Work out the finished part from the listing and answer in its coordinate system (mm). Face numbers are marked on the shaded views. A direction names the side the tool comes from. Round coordinates to 2 decimals unless told otherwise and drop trailing zeros. Loops run counter-clockwise (first coordinate to the right, second up) from the corner with the lowest first, then second, coordinate; pieces in that order, holes last. Notation, with made-up numbers: M 28.5,-11 L 67.5,-11 A24 ccw 67.5,21 Z; hole C -36,-35 d11. An arc over 180 degrees is marked long. One line per item, written item: value.
Autodesk Inventor part; units mm, degrees
ref_plane "YZ Plane" through (0, 0, 0) normal (1, 0, 0) x (0, 1, 0)
ref_plane "XZ Plane" through (0, 0, 0) normal (0, 1, 0) x (-1, 0, 0)
ref_plane "XY Plane" through (0, 0, 0) normal (0, 0, 1) x (1, 0, 0)
sketch "Sketch1" plane through (0, 0, 0) normal (0, 1, 0) x (-1, 0, 0)
  circle A0 centre (0, 0) radius 10
  circle A1 centre (0, 0) radius 8.6
extrude "Extrusion1" add sketch "Sketch1" along normal blind 5 contours A0 | A1
sketch "Sketch2" plane through (0, 0, 0) normal (0, -1, 0) x (1, 0, 0)
  circle A0 centre (0, 0) radius 8.6
  circle A1 centre (0, 0) radius 2.5
extrude "Extrusion2" add sketch "Sketch2" along normal blind 20 contours A0 | A1
sketch "Sketch3" plane through (0, -20, 0) normal (0, -1, 0) x (1, 0, 0)
  circle A0 centre (0, 0) radius 2.5
extrude "Extrusion3" cut sketch "Sketch3" against normal blind 10
sketch "Sketch4" plane through (0, 5, 0) normal (0, 1, 0) x (1, 0, 0)
  circle A0 centre (0, 0) radius 5
extrude "Extrusion4" add sketch "Sketch4" along normal blind 43
fillet "Fillet1" radius 2 1 edges at (-5, 48, 0)
properties part number "driven_shaft" material "Gold"
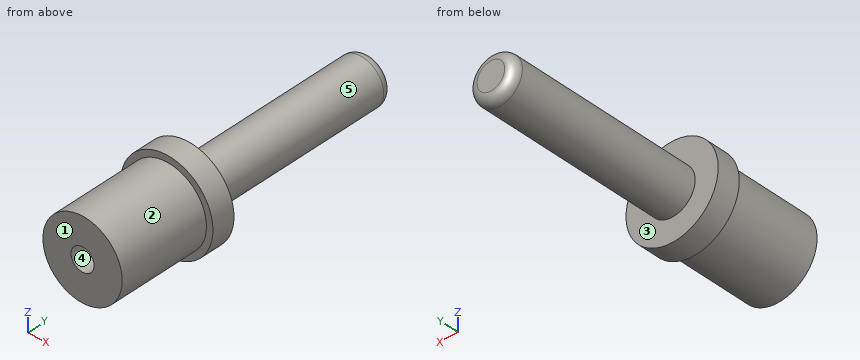
1) Find section A-A (z = 0). Give the vertices of the cut face in (x, y).
Check values:
outline: M -10,0 L -8.6,0 L -8.6,-20 L -2.5,-20 L -2.5,-10 L 2.5,-10 L 2.5,-20 L 8.6,-20 L 8.6,0 L 10,0 L 10,5 L 5,5 L 5,46 A2 ccw 3,48 L -3,48 A2 ccw -5,46 L -5,5 L -10,5 Z
2) Find section B-B (x = 0). Give the vertices of the cut face in (y, z).
Check values:
outline: M -20,-8.6 L 0,-8.6 L 0,-10 L 5,-10 L 5,-5 L 46,-5 A2 ccw 48,-3 L 48,3 A2 ccw 46,5 L 5,5 L 5,10 L 0,10 L 0,8.6 L -20,8.6 L -20,2.5 L -10,2.5 L -10,-2.5 L -20,-2.5 Z
3) For the marked faces 1 and 2, determine the directions among +Z, -Z, +X, -X, +Y, -Y from which every point of the face is accessible in a straight line to the end or side of a thin tool.
Check values:
face 1: +Z, -Z, +X, -X, -Y
face 2: -Y
4) The mould has two halves that part along X. Classify the marked faces 3, 4 and 5: +X half, -X half, draft (parallel to the pull), parting line (faces both ways), or undercut.
Check values:
face 3: draft
face 4: undercut
face 5: parting line
5) Each of these flat-tipped pins is pushed along its axis until it touches: pin 1 (1.5 mm diameter, centred on x = 1.5, y = 37.5, fed in from -Z); pin 2 (6 mm diameter, centred on y = 15, z = -3.5, fed in from -X); pin 3 (2 mm diameter, centred on x = -5.5, y = 14, fed in from -Z). Where does it stop, or does it pass through?
Check values:
pin 1: z = -4.94
pin 2: x = -4.97
pin 3: z = -2.18
6) Find section C-C (y = 12). Give the vertices of the cut face in (x, z), then the cut area to 3 significant figures.
Check values:
outline: C 0,0 d10
area: 78.5 mm2
7) Find section D-D (z = -5.75). Give the vertices of the cut face in (x, y).
Check values:
outline: M -8.18,0 L -6.4,0 L -6.4,-20 L 6.4,-20 L 6.4,0 L 8.18,0 L 8.18,5 L -8.18,5 Z
8) Find the intervals of material crossed by probe 1 along Z at (x, y) = (0, -15.5); probe 2 along Y at (x, z) = (0.75, 1.25); probe 3 along Y at (x, z) = (8, 3.5), in increasing order. Write a range as from..to.
Check values:
probe 1: -8.6..-2.5, 2.5..8.6
probe 2: -10..48
probe 3: 0..5
